Read the model definition and answer for the solid it produces. Units are mm, in the model's axes. Give positions to 0.01 mm unless a question says otherwise; leave off trailing zeros. Write each loop counter-clockwise with the first axis right and the second up, starting at its lowest first coordinate (ties: lowest second). Pieces come first, ordered by that corner, then holes. Notation, with made-up numbers: M 87,1.25 L 140,1.25 A12 cw 140,23.25 Z; hole C 7.25,-38.75 d9. An arc over 180 degrees is marked long. Use a Markdown table: item, result. Add a question column.
Item 1: A cutting plane is placed at C-C on z = -117.5. Determine the outline of the cut face in (x, y).
Item 2: Consider probe 1 along Y at (x, z) = (-85.75, 145); probe 2 along X at (y, z) = (278.25, -61); probe 3 along X at (y, z) = (263.5, -48.5). Determine where each line is inside the solid, lowest interval first. Write a range as [from, to].
Item 3: Given P1, Ø8, axis at x = -82, y = 280.5, coming from the -Z side; P2, Ø1, axis at y = 277.5, z = 94.5, coming from the +X side; P3, Ø3, axis at x = -78.5, y = 275, coming from the +Z side; P4, Ø12, axis at x = -88.5, z = -9.5, coming from the +Y side, each flat-ended and moving along its own axis, determine where each tip first touches the part or whether it passes through.
Item 4: A cutting plane is placed at A-A on y = 277.5. Determine the outline of the cut face in (x, z) (3 decimals).
Item 5: A cutting plane is placed at B-B on x = -92.75. Determine the outline of the cut face in (y, z) (3 decimals), then the cut area to 3 significant figures.
from build123d import *

# Parameters (mm, degrees)
SKETCH1_R           = 10.922
BOSS_EXTRUDE1_DEPTH = 161.925


with BuildPart() as part:
    # Sketch1 → Boss-Extrude1 (new body, symmetric)
    with BuildSketch(Plane.XY):
        with Locations((-85.411167397, 272.8722)):
            Circle(SKETCH1_R)
    extrude(amount=BOSS_EXTRUDE1_DEPTH, both=True)

    # Sketch3 → Revolve2 (revolve)
    with BuildSketch(Plane(origin=(0, 0, -161.925), x_dir=(-1, 0, 0), z_dir=(0, 0, -1))):
        with BuildLine():
            Line((74.489167397, 272.8722), (96.333167397, 272.8722))
            ThreePointArc((96.333167397, 272.8722), (85.411167397, 283.7942), (74.489167397, 272.8722))
        make_face()
    revolve(axis=Axis((-74.489167397, 272.8722, -161.925), (-1, 0, 0)))

    # Sketch4 → Revolve3 (revolve)
    with BuildSketch(Plane.XY.offset(161.925)):
        with BuildLine():
            Line((-74.489167397, 272.8722), (-96.333167397, 272.8722))
            ThreePointArc((-96.333167397, 272.8722), (-85.411167397, 283.7942), (-74.489167397, 272.8722))
        make_face()
    revolve(axis=Axis((-74.489167397, 272.8722, 161.925), (-1, 0, 0)))


solid = part.part
Filled in:
| question | item | result |
|---|---|---|
| 1 | outline | C -85.41,272.87 d21.84 |
| 2 | probe 1 | [261.96, 283.79] |
| 2 | probe 2 | [-94.92, -75.9] |
| 2 | probe 3 | [-91.02, -79.8] |
| 3 | P1 | z = -171.94 |
| 3 | P2 | x = -75.3 |
| 3 | P3 | z = 171.22 |
| 3 | P4 | y = 283.79 |
| 4 | outline | M -95.304,-161.925 A9.893 ccw -75.518,-161.925 L -75.518,161.925 A9.893 ccw -95.304,161.925 Z |
| 5 | outline | M 264.783,-161.925 A8.089 ccw 280.961,-161.925 L 280.961,161.925 A8.089 ccw 264.783,161.925 Z |
| 5 | area | 5,440 mm² |
